The listing builds one solid part. Answer for the finished solid, in the listing's coordinates (mm). Face numbers are marked on the shaded views. Coordinates: 2 decimals unless noted, no trailing zeros. Loops run counter-clockwise (first coordinate to the right, second up) from the corner with the lowest first, then second, coordinate; pieces in that order, holes last. Notation, with made-up numbers: M 17,56 L 72,56 A24 cw 72,86 Z; hole C -23,82 d8. An arc over 180 degrees is marked long. Answer as a JSON object with one key per item and string values. Group by question number.
1. Given pin 1 (3 mm diameter, centred on x = -0.5, z = 4.5, fed in from -Y); pin 2 (4 mm diameter, centred on x = 2.5, z = -4, fed in from +Y); pin 3 (1 mm diameter, centred on x = -3, z = 8.5, fed in from -Y), each flat-ended and moving along its own axis, determine where each tip first touches the part or whether it passes through.
2. Determine the mould class of the marked faces 1, 2 and 3 for opening direction Z: released by +Z, released by -Z, zero draft, split by the parting line, or undercut.
3. Straight lines are drawn through the part: L1, parallel to Z at x = 2, y = -3; L2, parallel to Y at x = 0, z = -3.25; L3, parallel to X at y = 1, z = 10.5. For each, find the intervals that lie inside material, in ascending order.
4. A cutting plane is placed at C-C on z = 3. Give the vertices of the cut face in (x, y), and give its area (3 significant figures).
5. A cutting plane is placed at A-A on x = 0. Give the vertices of the cut face in (y, z).
from build123d import *

# Parameters (mm, degrees)
SKETCH1_R           = 3.5
BOSS_EXTRUDE1_DEPTH = 12.5
SKETCH2_R           = 5
BOSS_EXTRUDE2_DEPTH = 1
CHAMFER1_SIZE       = 0.75


with BuildPart() as part:
    # Sketch1 → Boss-Extrude1 (new body, symmetric)
    with BuildSketch(Plane.XY):
        Circle(SKETCH1_R)
    extrude(amount=BOSS_EXTRUDE1_DEPTH, both=True)

    # Sketch2 → Boss-Extrude2 (add)
    with BuildSketch(Plane.XY.offset(12.5)):
        Circle(SKETCH2_R)
    boss_extrude2 = extrude(amount=BOSS_EXTRUDE2_DEPTH)

    # Mirror1: Boss-Extrude2 across plane
    add(boss_extrude2.mirror(Plane.XY))

    # Chamfer1
    chamfer1_edges = [part.edges().sort_by_distance(p)[0] for p in [
        (-5, 0, 13.5),
        (-5, 0, -13.5),
    ]]
    chamfer(chamfer1_edges, length=CHAMFER1_SIZE)


solid = part.part
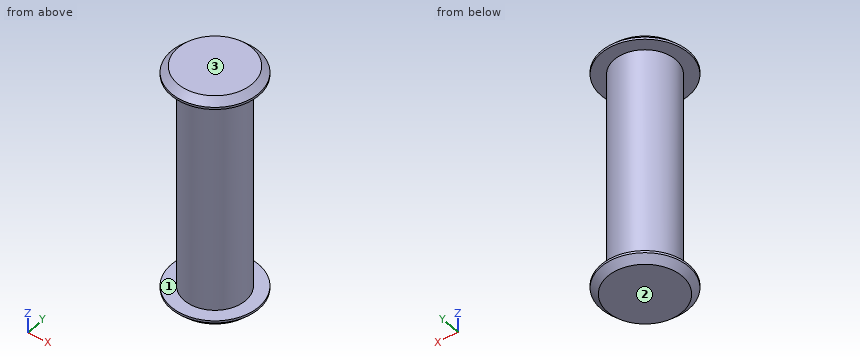
From the geometry:
{
 "1": {"pin 1": "stops at y = -3.5", "pin 2": "stops at y = 3.46", "pin 3": "stops at y = -2.45"},
 "2": {"face 1": "undercut", "face 2": "released by -Z", "face 3": "released by +Z"},
 "3": {"L1": "z = -13.5 to -12.5, 12.5 to 13.5", "L2": "y = -3.5 to 3.5", "L3": "x = -3.35 to 3.35"},
 "4": {"outline": "C 0,0 d7", "area": "38.5 mm²"},
 "5": {"outline": "M -5,-12.75 L -4.25,-13.5 L 4.25,-13.5 L 5,-12.75 L 5,-12.5 L 3.5,-12.5 L 3.5,12.5 L 5,12.5 L 5,12.75 L 4.25,13.5 L -4.25,13.5 L -5,12.75 L -5,12.5 L -3.5,12.5 L -3.5,-12.5 L -5,-12.5 Z"}
}
